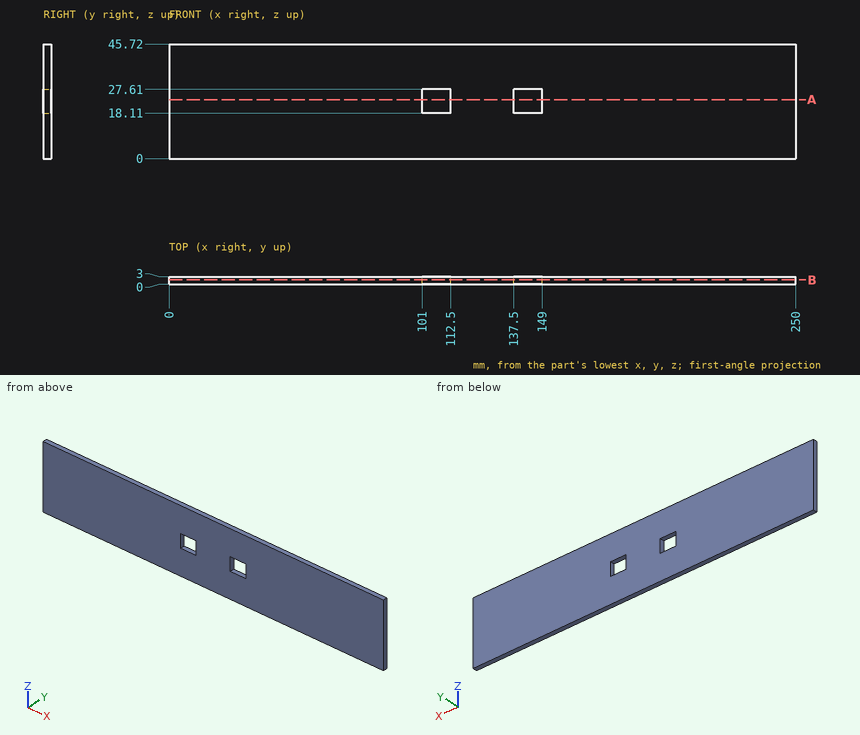
Study the drawing (mm; zero at the part's minimum x, y, z) and answer. Give positions to 0.01 mm unless a question says otherwise; leave off trailing zeros. Loops run counter-clockwise (first coordinate to the right, second up) from the corner with the lowest first, then second, coordinate; pieces in that order, holes last. Notation, with made-up numbers: (32.25, 49) -> (53.25, 49) arc R19 cw to (53.25, 74) -> close; hole circle Ø3 at (64, 63.5). An arc over 180 degrees is marked (long way). Use a Markdown table: item, result. Add a question column.
1) The part is cut by section B-B, the plane y = 1.7. Determine the outline of the cut face in (x, z), plus the area to 3 significant figures.
2) The part is cut by section A-A, the plane z = 23.5. Determine the outline of the cut face in (x, y), plus the area to 3 significant figures.
3) Consider line 1 along X through (y, z) = (0.55, 23). Determine where the line is inside the solid, lowest interval first.
Reported:
| question | item | result |
|---|---|---|
| 1 | outline | (0, 0) -> (250, 0) -> (250, 45.72) -> (0, 45.72) -> close; hole (101, 18.11) -> (112.5, 18.11) -> (112.5, 27.61) -> (101, 27.61) -> close; hole (137.5, 18.11) -> (149, 18.11) -> (149, 27.61) -> (137.5, 27.61) -> close |
| 1 | area | 11,200 mm^2 |
| 2 | outline | (0, 0) -> (101, 0) -> (101, 3) -> (0, 3) -> close; (112.5, 0) -> (137.5, 0) -> (137.5, 3) -> (112.5, 3) -> close; (149, 0) -> (250, 0) -> (250, 3) -> (149, 3) -> close |
| 2 | area | 681 mm^2 |
| 3 | line 1 | x = 0 to 101, 112.5 to 137.5, 149 to 250 |
